Read the model definition and answer for the solid it produces. Units are mm, in the model's axes. A direction names the side the tool comes from. Give positions to 0.01 mm unless a question says otherwise; leave off trailing zeros. Write each loop counter-clockwise with the first axis right and the second up, starting at its lowest first coordinate (ties: lowest second). Pieces come first, ordered by that corner, then holes. Notation, with made-up numbers: (82, -38.75) -> (138, -38.75) arc R29 cw to (138, -9.75) -> close; hole circle Ø5 at (40.5, -31). An arc over 180 degrees is marked (long way). Put each result on its own line as item: value. Start each with the question number.
from build123d import *

# Parameters (mm, degrees)
ESQUISSE1_R                  = 11
ESQUISSE1_R_2                = 4.5
ESQUISSE1_R_3                = 2.1
BOSS_EXTRU_1_DEPTH           = 5
BOSS_EXTRU_2_DEPTH           = 5
R_P_TITION_CIRCULAIRE1_COUNT = 37


with BuildPart() as part:
    # Esquisse1 → Boss.-Extru.1 (new body)
    with BuildSketch(Plane.XY):
        Circle(ESQUISSE1_R)
        Circle(ESQUISSE1_R_2, mode=Mode.SUBTRACT)
        with Locations((-5.5, 5.5)):
            Circle(ESQUISSE1_R_3, mode=Mode.SUBTRACT)
        with Locations(Location((5.5, -5.5, 0), (0, 0, 180))):
            Circle(ESQUISSE1_R_3, mode=Mode.SUBTRACT)
    extrude(amount=BOSS_EXTRU_1_DEPTH)

    # Esquisse2 → Boss.-Extru.2 (add)
    with BuildSketch(Plane.XY.offset(5)):
        Polygon((0, 12.892709197), (-0.883743736, 10.692594879), (0.883743736, 10.692594879), align=None)
    boss_extru_2 = extrude(amount=-BOSS_EXTRU_2_DEPTH)

    # Répétition circulaire1: Boss.-Extru.2 ×37 about axis
    r_p_tition_circulaire1_axis = Axis((0, 0, 0), (0, 0, 1))
    for i in range(1, R_P_TITION_CIRCULAIRE1_COUNT):
        add(boss_extru_2.rotate(r_p_tition_circulaire1_axis, i * 360 / R_P_TITION_CIRCULAIRE1_COUNT))


solid = part.part
1) Each of these flat-tipped pins is pushed along its axis until it touches: pin 1 Ø2 at (x, z) = (5.5, 4.5) entering from -Y; pin 2 Ø1 at (x, z) = (-10.5, 1.5) entering from +Y; pin 3 Ø3 at (x, z) = (10, 3) entering from -Y; pin 4 Ø12 at (x, y) = (9.5, -8.5) entering from +Z. Where does it stop, or does it pass through?
2) For faces 4 (the face through (9.83, -6.8, 2.54)), 5 (the face through (6.351, -10.094, 2.535)), 6 (the face through (-0.4, 11.9, 2.5)), 7 (the face through (-11.511, -3.116, 2.535)), 8 (the face through (5.267, -10.729, 2.535)), determine the directions among +Z, -Z, +X, -X, +Y, -Y from which every point of the face is accessible in a straight line to the end or side of a thin tool.
3) Straight lines are drawn through the part: line 1 (X direction, y = -1.25, z = 2.3); line 2 (Y direction, x = 5.5, z = 2.8); line 3 (X direction, y = -8.75, z = 0.4). For each, find the intervals that lie inside material, in ascending order. Write a range as [from, to].
4) A cutting plane is placed at C-C on z = 2.5. State how many separate pieces and enclosed holes the cut face has, and give its area (3 significant figures).
5) A cutting plane is placed at A-A on y = 0. Give the vertices of the cut face in (x, z).
6) A cutting plane is placed at B-B on y = 4. Give the vertices of the cut face in (x, z), and give its area (3 significant figures).
7) For a pull along Y with two mould halves and no side action, classify faces 1 (the face through (-0.634, -11.935, 2.535)), 2 (the face through (-8.53, -8.335, 2.535)), 3 (the face through (-5.472, 10.596, 2.535)) as pulls with the +Y half, pulls with the -Y half, needs draft (parallel to the pull), parting line crosses it, or undercut.
Results found:
1. pin 1: stops at y = -11.75
1. pin 2: stops at y = 6.76
1. pin 3: stops at y = -9.31
1. pin 4: stops at z = 5
2. face 4: +Z, -Z, +X
2. face 5: +Z, -Z, -Y
2. face 6: +Z, -Z, +Y
2. face 7: +Z, -Z, -X
2. face 8: +Z, -Z
3. line 1: x = [-12.09, -4.32], [4.32, 12.09]
3. line 2: y = [-9.53, -7.6], [-3.4, 10.62]
3. line 3: x = [-8.7, -7.69], [-6.8, 6.8], [7.69, 8.7]
4. separate pieces: 1
4. enclosed holes: 3
4. area: 343 mm²
5. outline: (-11.67, 0) -> (-4.5, 0) -> (-4.5, 5) -> (-11.67, 5) -> close; (4.5, 0) -> (11.67, 0) -> (11.67, 5) -> (4.5, 5) -> close
6. outline: (-11.12, 0) -> (-6.97, 0) -> (-6.97, 5) -> (-11.12, 5) -> close; (-4.03, 0) -> (-2.06, 0) -> (-2.06, 5) -> (-4.03, 5) -> close; (2.06, 0) -> (11.12, 0) -> (11.12, 5) -> (2.06, 5) -> close
6. area: 75.9 mm²
7. face 1: pulls with the -Y half
7. face 2: undercut
7. face 3: pulls with the +Y half
